```python
from build123d import *

# Parameters (mm, degrees)
ESQUISSE1_W             = 130
ESQUISSE1_H             = 45
BOSS_EXTRU_1_DEPTH      = 6.35
ENL_V_MAT_EXTRU_1_REACH = 81.312
ESQUISSE3_W             = 25
ESQUISSE3_H             = 6.35
BOSS_EXTRU_2_DEPTH      = 6.35


with BuildPart() as part:
    # Esquisse1 → Boss.-Extru.1 (new body)
    with BuildSketch(Plane.XY):
        with Locations((0, 22.5)):
            Rectangle(ESQUISSE1_W, ESQUISSE1_H)
    extrude(amount=BOSS_EXTRU_1_DEPTH)

    # Esquisse2 → Enlèv. mat.-Extru.1 (cut, up to next)
    with BuildSketch(Plane.XY.offset(6.35), mode=Mode.PRIVATE) as enl_v_mat_extru_1_sk1:
        with BuildLine():
            Line((-47, 35), (-18, 35))
            ThreePointArc((-18, 35), (-5.5, 22.5), (-18, 10))
            Line((-18, 10), (-47, 10))
            ThreePointArc((-47, 10), (-59.5, 22.5), (-47, 35))
        make_face()
    enl_v_mat_extru_1_tool1 = extrude(enl_v_mat_extru_1_sk1.sketch, amount=-ENL_V_MAT_EXTRU_1_REACH, mode=Mode.PRIVATE) & part.part
    # Esquisse2 → Enlèv. mat.-Extru.1 (cut, up to next)
    with BuildSketch(Plane.XY.offset(6.35), mode=Mode.PRIVATE) as enl_v_mat_extru_1_sk2:
        with BuildLine():
            Line((47, 35), (18, 35))
            ThreePointArc((18, 35), (5.5, 22.5), (18, 10))
            Line((18, 10), (47, 10))
            ThreePointArc((47, 10), (59.5, 22.5), (47, 35))
        make_face()
    enl_v_mat_extru_1_tool2 = extrude(enl_v_mat_extru_1_sk2.sketch, amount=-ENL_V_MAT_EXTRU_1_REACH, mode=Mode.PRIVATE) & part.part
    add(enl_v_mat_extru_1_tool1.solids().sort_by_distance((-32.5, 22.5, 6.35))[0], mode=Mode.SUBTRACT)
    add(enl_v_mat_extru_1_tool2.solids().sort_by_distance((32.5, 22.5, 6.35))[0], mode=Mode.SUBTRACT)

    # Esquisse3 → Boss.-Extru.2 (add)
    with BuildSketch(Plane.XY.offset(6.35)):
        with Locations((-32.5, 48.175)):
            Rectangle(ESQUISSE3_W, ESQUISSE3_H)
        with Locations((-32.5, -3.175)):
            Rectangle(ESQUISSE3_W, ESQUISSE3_H)
        with Locations((32.5, 48.175)):
            Rectangle(ESQUISSE3_W, ESQUISSE3_H)
        with Locations((32.5, -3.175)):
            Rectangle(ESQUISSE3_W, ESQUISSE3_H)
    extrude(amount=-BOSS_EXTRU_2_DEPTH)


solid = part.part
```
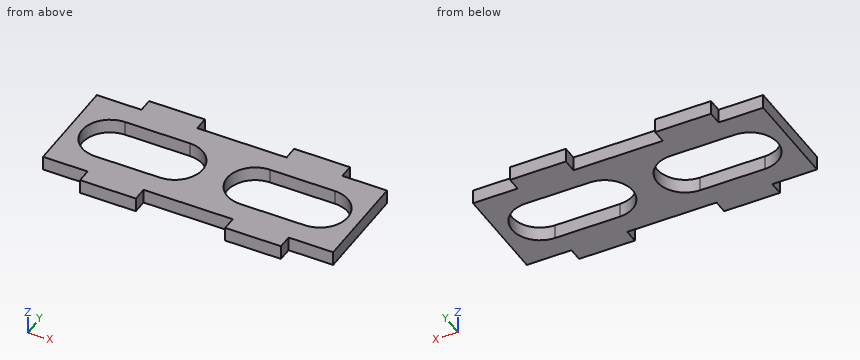
Part model, mm, in its own coordinate system. Coordinates: 2 decimals unless noted, no trailing zeros. Write each loop counter-clockwise with the first axis right and the second up, starting at its lowest first coordinate (ties: lowest second). Pieces come first, ordered by that corner, then holes.
Item 1: Slice it at D-D (y = 22.5). Write the cut outline in (x, z).
Item 2: Slice it at B-B (x = 29). Write the cut outline in (y, z).
Item 3: Probe line 1 (Y direction, x = 19.5, z = 2.5); line 2 (Y direction, x = 34, z = 6.25); line 3 (X direction, y = 26.5, z = 5). List the from-to ranges inside material, lowest first.
Item 4: Pin check, flat tips, straight feed: pin 1 (1.9 mm diameter, centred on x = -10, z = 3.5, fed in from +Y); pin 2 (3 mm diameter, centred on x = 58, z = 3.5, fed in from -Y); pin 3 (3 mm diameter, centred on y = 49, z = 1.5, fed in from +X). Stop position of each tip, or through.
Item 5: Slice it at A-A (y = 30). Write the cut outline in (x, z), and give its area (3 significant figures).
Item 6: Slice it at C-C (z = 3.25). Write the cut outline in (x, y), and give its area (3 significant figures).
Results found:
1. outline: (-65, 0) - (-59.5, 0) - (-59.5, 6.35) - (-65, 6.35) - close; (-5.5, 0) - (5.5, 0) - (5.5, 6.35) - (-5.5, 6.35) - close; (59.5, 0) - (65, 0) - (65, 6.35) - (59.5, 6.35) - close
2. outline: (-6.35, 0) - (10, 0) - (10, 6.35) - (-6.35, 6.35) - close; (35, 0) - (51.35, 0) - (51.35, 6.35) - (35, 6.35) - close
3. line 1: y = 0 to 10, 35 to 45
3. line 2: y = -6.35 to 10, 35 to 51.35
3. line 3: x = -65 to -58.84, -6.16 to 6.16, 58.84 to 65
4. pin 1: stops at y = 45
4. pin 2: stops at y = 0
4. pin 3: stops at x = 45
5. outline: (-65, 0) - (-57, 0) - (-57, 6.35) - (-65, 6.35) - close; (-8, 0) - (8, 0) - (8, 6.35) - (-8, 6.35) - close; (57, 0) - (65, 0) - (65, 6.35) - (57, 6.35) - close
5. area: 203 mm2
6. outline: (-65, 0) - (-45, 0) - (-45, -6.35) - (-20, -6.35) - (-20, 0) - (20, 0) - (20, -6.35) - (45, -6.35) - (45, 0) - (65, 0) - (65, 45) - (45, 45) - (45, 51.35) - (20, 51.35) - (20, 45) - (-20, 45) - (-20, 51.35) - (-45, 51.35) - (-45, 45) - (-65, 45) - close; hole (-47, 10) - (-18, 10) arc R12.5 ccw to (-18, 35) - (-47, 35) arc R12.5 ccw to start; hole (18, 10) - (47, 10) arc R12.5 ccw to (47, 35) - (18, 35) arc R12.5 ccw to start
6. area: 4,050 mm2
